from build123d import *

# Parameters (mm, degrees)
EXTRUDE_1_DEPTH = 25
SKETCH_2_W      = 80
SKETCH_2_H      = 80
EXTRUDE_2_DEPTH = 10


with BuildPart() as part:
    # 草图1 → 凸台-拉伸1 (new body, symmetric)
    with BuildSketch(Plane.XY):
        Polygon((-350, 0), (-350, 550), (350, 550), (350, 0), (300, 0), (300, 500), (-300, 500), (-300, 0), align=None)
    extrude(amount=EXTRUDE_1_DEPTH, both=True)

    # 草图2 → 凸台-拉伸2 (add)
    with BuildSketch(Plane.XZ):
        with Locations((-325, 0)):
            Rectangle(SKETCH_2_W, SKETCH_2_H)
        with Locations((325, 0)):
            Rectangle(SKETCH_2_W, SKETCH_2_H)
    extrude(amount=EXTRUDE_2_DEPTH)


solid = part.part
The listing builds one solid part. Answer for the finished solid, in the listing's coordinates (mm). A direction names the side the tool comes from. Give positions to 0.01 mm unless a question says otherwise; leave off trailing zeros. Loops run counter-clockwise (first coordinate to the right, second up) from the corner with the lowest first, then second, coordinate; pieces in that order, holes last. Notation, with made-up numbers: M 37.5,33 L 46.5,33 A6 cw 46.5,38 Z; hole C 0,74.5 d1. An arc over 180 degrees is marked long. Answer as CSV lines item,"result".
Item 1: The mould has two halves that part along X. Classify faces 4 (the flat face through (4, 500, 0)), 5 (the flat face through (350, 279, 0)), 6 (the flat face through (324, -10, 1)), 7 (the flat face through (300, 247, 0)): released by +X, released by -X, zero draft, split by the parting line, or undercut.
Values follow:
face 4,"undercut"
face 5,"released by +X"
face 6,"zero draft"
face 7,"undercut"
Item 2: The part is cut by section B-B (z = -15.5). Give the vertices of the cut face in (x, y).
Values follow:
outline,"M -365,-10 L -285,-10 L -285,0 L -300,0 L -300,500 L 300,500 L 300,0 L 285,0 L 285,-10 L 365,-10 L 365,0 L 350,0 L 350,550 L -350,550 L -350,0 L -365,0 Z"
Item 3: The part is cut by section C-C (x = 257). Give the vertices of the cut face in (y, z).
Values follow:
outline,"M 500,-25 L 550,-25 L 550,25 L 500,25 Z"
Item 4: Which of the six approach directions +Z, -Z, +X, -X, +Y, -Y give full straight-line access (tool end or side, diameter ignored) to faces 1 (the flat face through (1.6, 500.4, -25)), 2 (the flat face through (-350, 271, 0)), 3 (the flat face through (351, 0, 1))?
Values follow:
face 1,"-Z, +X, -X, +Y"
face 2,"+Z, -Z, -X, +Y"
face 3,"none"
Item 5: Given pin 1 Ø15 at (y, z) = (205, -7.5) entering from +X; pin 2 Ø1 at (x, z) = (-174.5, -17) entering from -Y; pin 3 Ø5 at (y, z) = (447, 0.5) entering from -X, each flat-ended and moving along its own axis, determine where each tip first touches the part or whether it passes through.
Values follow:
pin 1,"stops at x = 350"
pin 2,"stops at y = 500"
pin 3,"stops at x = -350"
Item 6: The part is cut by section A-A (y = 214.5). Give the vertices of the cut face in (x, z).
Values follow:
outline,"M -350,-25 L -300,-25 L -300,25 L -350,25 Z; M 300,-25 L 350,-25 L 350,25 L 300,25 Z"
Item 7: Straight lines are drawn through the part: line 1 along X through (y, z) = (466.5, 21); line 2 along Z through (x, y) = (-323.5, 455); line 3 along Y through (x, z) = (204.5, 4.5). For each, find the intervals that lie inside material, in ascending order. Write a range as [from, to].
Values follow:
line 1,"x = [-350, -300], [300, 350]"
line 2,"z = [-25, 25]"
line 3,"y = [500, 550]"
